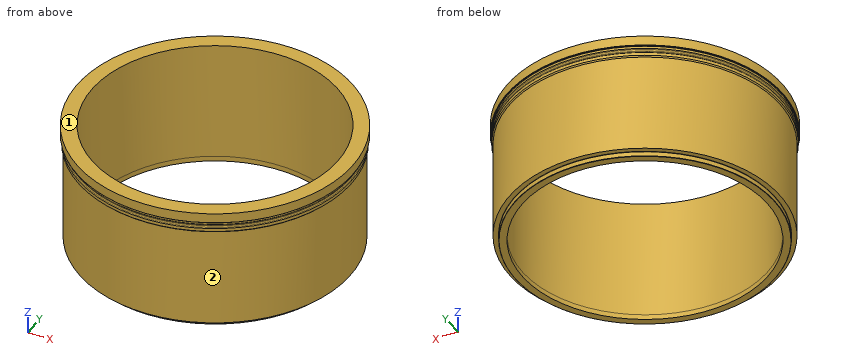
Autodesk Inventor part; units mm, degrees
ref_plane "YZ Plane" through (0, 0, 0) normal (1, 0, 0) x (0, 1, 0)
ref_plane "XZ Plane" through (0, 0, 0) normal (0, 1, 0) x (-1, 0, 0)
ref_plane "XY Plane" through (0, 0, 0) normal (0, 0, 1) x (1, 0, 0)
sketch "Sketch1" plane through (0, 0, 0) normal (0, 0, 1) x (1, 0, 0)
  circle A0 centre (0, 0) radius 311.15
  circle A1 centre (0, 0) radius 342.9
  dimension "d0" = 622.3
  dimension "d1" = 685.8
extrude "Extrusion1" add sketch "Sketch1" along normal blind 304.8
sketch "Sketch2" plane through (0, 0, 304.8) normal (0, 0, 1) x (1, 0, 0)
  circle A0 centre (0, 0) radius 342.9
  circle A1 centre (0, 0) radius 345.821
  circle A2 centre (0, 0) radius 348.996
  dimension "d4" = 691.642
  dimension "d5" = 697.992
extrude "Extrusion2" add sketch "Sketch2" against normal blind 50.8 contours A1
extrude "Extrusion3" add sketch "Sketch2" against normal blind 25.4 contours A2
chamfer "Chamfer1" distance 2.921 angle 45 1 edges at (-342.9, 0, 254)
sketch "Sketch3" plane through (0, 0, 0) normal (0, 0, -1) x (-1, 0, 0)
  circle A0 centre (0, 0) radius 329.946
  circle A1 centre (0, 0) radius 311.15
  dimension "d13" = 659.892
extrude "Extrusion4" add sketch "Sketch3" along normal blind 12.7
fillet "Fillet1" radius 0.7937 2 edges at (329.946, 0, 0) (-345.821, 0, 279.4)
chamfer "Chamfer2" distance 0.7937 angle 45 1 edges at (329.946, 0, -12.7)
chamfer "Chamfer3" distance 0.7937 angle 45 1 edges at (-348.996, 0, 279.4)
sketch "Sketch4" plane through (0, 0, 0) normal (1, 0, 0) x (0, 1, 0)
  line L0 (345.821, 278.6062) -> (345.821, 254) construction
  line L1 (-348.996, 304.8) -> (348.996, 304.8) construction
  line L2 (345.821, 273.05) -> (344.0409, 271.2699)
  arc A0 (344.0409, 271.2699) -> (342.646, 267.9023) centre (347.4085, 267.9023) ccw
  line L3 (342.646, 267.9023) -> (342.646, 267.0852)
  arc A1 (342.646, 267.0852) -> (344.0409, 263.7176) centre (347.4085, 267.0852) ccw
  line L4 (344.0409, 263.7176) -> (345.821, 261.9375)
  line L5 (345.821, 261.9375) -> (345.821, 273.05)
  line L6 (0, -60.96) -> (0, 365.76)
  point P0 (0, 0)
  dimension "d23" = 11.1125
  dimension "d24" = 3.175
  dimension "d25" = 4.7625
  dimension "d26" = 31.75
  dimension "d27" = 45
revolve "Revolution1" cut sketch "Sketch4" angle 360 about axis through (0, 0, -10) along (0, 0, 1)
equation "\"d10\" = -0.5 * d1 + 0.5 * d4"
properties part number "A1-19037-300-06 HCWI liner - pup" material "Iron, HCWI"
Check sheet for the modelled part. Datum: model origin and axes. Units: mm. Face numbers are marked on the shaded views. A direction names the side the tool comes from. Coordinates: 2 decimals unless noted, no trailing zeros. Loops run counter-clockwise (first coordinate to the right, second up) from the corner with the lowest first, then second, coordinate; pieces in that order, holes last.
1) Sectioned sample at A-A (z = 138.5). Record the boundary of the cut face in (x, y), and give its area (3 significant figures).
2) Material ranges on probe 1 along Y at (x, z) = (0, 203); probe 2 along Y at (x, z) = (0, -6); probe 3 along Z at (x, y) = (295, 153), recorded low to high.
3) Gauge pin test, flat ends, axial feed: pin 1 (10 mm diameter, centred on x = -205, y = 273.5, fed in from -Z); pin 2 (1 mm diameter, centred on x = -220.5, z = 171, fed in from -Y); pin 3 (5 mm diameter, centred on x = -150, z = 206.5, fed in from +Y). Record the tip position at first contact, or that the pin passes through.
4) Access from +Z, -Z, +X, -X, +Y, -Y to the whole of each face (thin tool, end or side, straight path). Record for the marked faces 1 and 2.
Check sheet entries:
1. outline: circle Ø685.8 at (0, 0); hole circle Ø622.3 at (0, 0)
1. area: 65,200 mm2
2. probe 1: y = -342.9 to -311.15, 311.15 to 342.9
2. probe 2: y = -329.95 to -311.15, 311.15 to 329.95
2. probe 3: z = 0 to 304.8
3. pin 1: stops at z = 0
3. pin 2: stops at y = -263.02
3. pin 3: stops at y = 309.55
4. face 1: +Z, +X, -X, +Y, -Y
4. face 2: -Z
